Input: part model. Units: mm. Frame: model coordinates. A direction names the side the tool comes from. Round coordinates to 2 decimals unless told otherwise and drop trailing zeros. Loops run counter-clockwise (first coordinate to the right, second up) from the corner with the lowest first, then second, coordinate; pieces in that order, holes last. Notation, with made-up numbers: (-3.75, 14) -> (8.25, 14) arc R11 cw to (8.25, 34) -> close; hole circle Ø11 at (-18.75, 73). An arc over 180 degrees is marked (long way). Answer as a JSON object with one key per item and string values. Group by question number.
Item 1: Section query A-A on y = -34. Return loops of the section in (x, z), and give its area (3 significant figures).
Item 2: Section query B-B on x = -19.5. Return loops of the section in (y, z), and give its area (3 significant figures).
Item 3: Set-up query: faces 1 (the flat face through (-21, -21, 54)), 2 (the cylindrical face through (-22, -25, 84)), 3 (the cylindrical face through (-28.538, -20.115, 27.507)), 4 (the flat face through (-31.963, -34.137, 65.479)). Return all of +Z, -Z, +X, -X, +Y, -Y with unobstructed straight access to the full face (end or side cutting, diameter ignored); none if empty.
Item 4: Pin query (flat end, axial travel): pin 1 (1.5 mm diameter, centred on x = -23, y = -18, fed in from -Z); pin 2 (2 mm diameter, centred on x = -28, y = -21, fed in from -Z); pin 3 (1 mm diameter, centred on y = -23.5, z = 30.5, fed in from +X); pin 4 (6.5 mm diameter, centred on x = -25, y = -27, fed in from -Z). Return the tip coordinate at first contact, or that it passes through.
Item 5: Section query C-C on z = 68.5. Return loops of the section in (x, y).
Item 6: Material intervals for line 1 (Z direction, x = -18.25, y = -26.5); line 2 (Z direction, x = -30.25, y = -31); line 3 (Z direction, x = -21.5, y = -21), sorted ascending. Write a range as [from, to].
Item 7: Section query D-D on y = -23. Return loops of the section in (x, z).
from build123d import *

# Parameters (mm, degrees)
SKETCH014_R             = 6
PAD012_DEPTH            = 7.5
SKETCH015_R             = 6.5
PAD013_DEPTH            = 42.5
SKETCH016_R             = 6
PAD014_DEPTH            = 10
SKETCH017_R             = 3
PAD015_DEPTH            = 6
SKETCH018_R             = 1
PAD016_DEPTH            = 1
PAD017_DEPTH            = 3
SKETCH020_R             = 7.741832
PAD018_DEPTH            = 10
PAD019_DEPTH            = 3
BODY003_PLACEMENT_ANGLE = 180


with BuildPart() as part:
    # Sketch014 → Pad012 (new body)
    with BuildSketch(Plane.XY):
        Circle(SKETCH014_R)
    extrude(amount=PAD012_DEPTH)

    # Sketch015 (on Face3 of Pad012) → Pad013 (join)
    with BuildSketch(Plane.XY.offset(7.5)):
        Circle(SKETCH015_R)
    extrude(amount=PAD013_DEPTH)

    # Sketch016 (on Face5 of Pad013) → Pad014 (join)
    with BuildSketch(Plane.XY.offset(50)):
        Circle(SKETCH016_R)
    extrude(amount=PAD014_DEPTH)

    # Sketch017 (on Face7 of Pad014) → Pad015 (join)
    with BuildSketch(Plane.XY.offset(60)):
        with Locations((0, -1.61854)):
            Circle(SKETCH017_R)
    extrude(amount=PAD015_DEPTH)

    # Sketch018 (on Face7 of Pad015) → Pad016 (join)
    with BuildSketch(Plane.XY.offset(60)):
        with Locations((0, 4.042031)):
            Circle(SKETCH018_R)
    extrude(amount=PAD016_DEPTH)

    # Sketch019 (on Face2 of Pad016) → Pad017 (join)
    with BuildSketch(Plane(origin=(0, 0, 24), x_dir=(1, 0, 0), z_dir=(0, 0, -1))):
        Polygon((0, 10.722278), (-7.738631, 7.406596), (-10.866129, -0.409983), (-7.550447, -8.148615), (0.266132, -11.276112), (8.004764, -7.960431), (11.132261, -0.143851), (7.81658, 7.59478), align=None)
    extrude(amount=PAD017_DEPTH)

    # Sketch020 (on Face14 of Pad017) → Pad018 (join)
    with BuildSketch(Plane.XY.offset(24)):
        Circle(SKETCH020_R)
    extrude(amount=PAD018_DEPTH)

    # Sketch021 (on Face16 of Pad018) → Pad019 (join)
    with BuildSketch(Plane.XY.offset(34)):
        Polygon((0, 11), (-7.778175, 7.778175), (-11, 0), (-7.778175, -7.778175), (0, -11), (7.778175, -7.778175), (11, 0), (7.778175, 7.778175), align=None)
    extrude(amount=PAD019_DEPTH)


with BuildPart() as part_1:
    # Body003 placement: moved
    add(part.part.moved(Location((-28, -25, 88))).rotate(Axis((-28, -25, 88), (0, 1, 0)), BODY003_PLACEMENT_ANGLE))


solid = part_1.part
Solved:
{
 "1": {"outline": "(-32.83, 51) -> (-23.17, 51) -> (-23.17, 54) -> (-32.83, 54) -> close; (-32.3, 64) -> (-23.98, 64) -> (-23.98, 67) -> (-32.3, 67) -> close", "area": "53.9 mm²"},
 "2": {"outline": "(-31.04, 51) -> (-18.96, 51) -> (-18.96, 54) -> (-31.04, 54) -> close; (-30.5, 64) -> (-19.07, 64) -> (-19.07, 67) -> (-30.5, 67) -> close", "area": "70.5 mm²"},
 "3": {"face 1": "none", "face 2": "+Z", "face 3": "-Z", "face 4": "+Z, -X, -Y"},
 "4": {"pin 1": "z = 51", "pin 2": "z = 27", "pin 3": "x = -22.08", "pin 4": "z = 22"},
 "5": {"outline": "circle Ø13 at (-28, -25)"},
 "6": {"line 1": "[51, 54], [64, 67]", "line 2": "[38, 80.5]", "line 3": "[51, 67]"},
 "7": {"outline": "(-38.39, 64) -> (-35.48, 64) -> (-35.48, 54) -> (-38.17, 54) -> (-38.17, 51) -> (-34.18, 51) -> (-34.18, 38) -> (-33.66, 38) -> (-33.66, 28) -> (-22.34, 28) -> (-22.34, 38) -> (-21.82, 38) -> (-21.82, 51) -> (-17.83, 51) -> (-17.83, 54) -> (-20.52, 54) -> (-20.52, 64) -> (-17.82, 64) -> (-17.82, 67) -> (-21.82, 67) -> (-21.82, 80.5) -> (-22.34, 80.5) -> (-22.34, 88) -> (-33.66, 88) -> (-33.66, 80.5) -> (-34.18, 80.5) -> (-34.18, 67) -> (-38.39, 67) -> close"}
}
